```python
from build123d import *

# Parameters (mm, degrees)
SKETCH2_R           = 262.5
SKETCH2_R_2         = 75
SKETCH2_R_3         = 3.2639
SKETCH2_R_4         = 3.25
BOSS_EXTRUDE1_DEPTH = 6.35


with BuildPart() as part:
    # Sketch2 → Boss-Extrude1 (new body)
    with BuildSketch(Plane(origin=(0, 0, 0), x_dir=(1, 0, 0), z_dir=(0, 1, 0))):
        with Locations(Location((0, 0, 0), (0, 0, 270))):
            Circle(SKETCH2_R)
        with Locations(Location((0, 0, 0), (0, 0, 270))):
            Circle(SKETCH2_R_2, mode=Mode.SUBTRACT)
        with Locations(Location((-232.5, 12.7, 0), (0, 0, 270))):
            Circle(SKETCH2_R_3, mode=Mode.SUBTRACT)
        with Locations(Location((-172.5, 12.7, 0), (0, 0, 270))):
            Circle(SKETCH2_R_3, mode=Mode.SUBTRACT)
        with Locations(Location((-112.5, 12.7, 0), (0, 0, 270))):
            Circle(SKETCH2_R_3, mode=Mode.SUBTRACT)
        with Locations(Location((112.5, 12.7, 0), (0, 0, 270))):
            Circle(SKETCH2_R_3, mode=Mode.SUBTRACT)
        with Locations(Location((172.5, 12.7, 0), (0, 0, 270))):
            Circle(SKETCH2_R_3, mode=Mode.SUBTRACT)
        with Locations(Location((232.5, 12.7, 0), (0, 0, 270))):
            Circle(SKETCH2_R_3, mode=Mode.SUBTRACT)
        with Locations(Location((232.5, -12.7, 0), (0, 0, 270))):
            Circle(SKETCH2_R_3, mode=Mode.SUBTRACT)
        with Locations(Location((172.5, -12.7, 0), (0, 0, 270))):
            Circle(SKETCH2_R_3, mode=Mode.SUBTRACT)
        with Locations(Location((112.5, -12.7, 0), (0, 0, 270))):
            Circle(SKETCH2_R_3, mode=Mode.SUBTRACT)
        with Locations(Location((-112.5, -12.7, 0), (0, 0, 270))):
            Circle(SKETCH2_R_3, mode=Mode.SUBTRACT)
        with Locations(Location((-172.5, -12.7, 0), (0, 0, 270))):
            Circle(SKETCH2_R_3, mode=Mode.SUBTRACT)
        with Locations(Location((-232.5, -12.7, 0), (0, 0, 270))):
            Circle(SKETCH2_R_3, mode=Mode.SUBTRACT)
        with Locations(Location((-173.205080757, 100, 0), (0, 0, 270))):
            Circle(SKETCH2_R_4, mode=Mode.SUBTRACT)
        with Locations(Location((173.205080757, 100, 0), (0, 0, 270))):
            Circle(SKETCH2_R_4, mode=Mode.SUBTRACT)
        with Locations(Location((0, -200, 0), (0, 0, 270))):
            Circle(SKETCH2_R_4, mode=Mode.SUBTRACT)
        with BuildLine():
            Line((-43.05, 236.77567), (-43.05, 161.77567))
            ThreePointArc((-43.05, 161.77567), (-45.55, 159.27567), (-48.05, 161.77567))
            Line((-48.05, 161.77567), (-48.05, 236.77567))
            ThreePointArc((-48.05, 236.77567), (-45.55, 239.27567), (-43.05, 236.77567))
        make_face(mode=Mode.SUBTRACT)
        with BuildLine():
            Line((43.05, 236.77567), (43.05, 161.77567))
            ThreePointArc((43.05, 161.77567), (45.55, 159.27567), (48.05, 161.77567))
            Line((48.05, 161.77567), (48.05, 236.77567))
            ThreePointArc((48.05, 236.77567), (45.55, 239.27567), (43.05, 236.77567))
        make_face(mode=Mode.SUBTRACT)
        with BuildLine():
            Line((226.578745218, -81.105441367), (161.626839934, -43.605441367))
            ThreePointArc((161.626839934, -43.605441367), (160.711776425, -40.190377858), (164.126839934, -39.275314348))
            Line((164.126839934, -39.275314348), (229.078745218, -76.775314348))
            ThreePointArc((229.078745218, -76.775314348), (229.993808728, -80.190377858), (226.578745218, -81.105441367))
        make_face(mode=Mode.SUBTRACT)
        with BuildLine():
            Line((183.528745218, -155.670228633), (118.576839934, -118.170228633))
            ThreePointArc((118.576839934, -118.170228633), (115.161776425, -119.085292142), (116.076839934, -122.500355652))
            Line((116.076839934, -122.500355652), (181.028745218, -160.000355652))
            ThreePointArc((181.028745218, -160.000355652), (184.443808728, -159.085292142), (183.528745218, -155.670228633))
        make_face(mode=Mode.SUBTRACT)
        with BuildLine():
            Line((-183.528745218, -155.670228633), (-118.576839934, -118.170228633))
            ThreePointArc((-118.576839934, -118.170228633), (-115.161776425, -119.085292142), (-116.076839934, -122.500355652))
            Line((-116.076839934, -122.500355652), (-181.028745218, -160.000355652))
            ThreePointArc((-181.028745218, -160.000355652), (-184.443808728, -159.085292142), (-183.528745218, -155.670228633))
        make_face(mode=Mode.SUBTRACT)
        with BuildLine():
            Line((-226.578745218, -81.105441367), (-161.626839934, -43.605441367))
            ThreePointArc((-161.626839934, -43.605441367), (-160.711776425, -40.190377858), (-164.126839934, -39.275314348))
            Line((-164.126839934, -39.275314348), (-229.078745218, -76.775314348))
            ThreePointArc((-229.078745218, -76.775314348), (-229.993808728, -80.190377858), (-226.578745218, -81.105441367))
        make_face(mode=Mode.SUBTRACT)
    extrude(amount=BOSS_EXTRUDE1_DEPTH)


solid = part.part
```
Geometry check sheet. Reference: the model listing, model coordinates, mm. A direction names the side the tool comes from. Round coordinates to 2 decimals unless told otherwise and drop trailing zeros. Order: outer loops, then holes, each group sorted by start corner. A loop starts at its lowest first (then second) coordinate and runs counter-clockwise, first axis right, second up. Notation, with made-up numbers: (37, 64.25) - (53, 64.25) arc R15 ccw to (53, 87.25) - close; hole circle Ø5 at (67.5, 47.5). An arc over 180 degrees is marked (long way). Use a Markdown table: item, result. Add a question column.
(1) Depth check by flat-ended pin: pin 1 (1.5 mm diameter, centred on y = 2.5, z = -195.5, fed in from -X); pin 2 (3 mm diameter, centred on y = 2, z = -211.5, fed in from +X); pin 3 (6 mm diameter, centred on x = -173.21, z = -100, fed in from -Y); pin 4 (1.9 mm diameter, centred on y = 2, z = -191.5, fed in from +X). Enter the tip coordinate at first touch or a pass-through.
(2) Material ranges on line 1 along Z through (x, y) = (-231, 2.5); line 2 along X through (y, z) = (1, -187.5); line 3 along X through (y, z) = (1.25, -212.5), recorded low to high. Write a range as [from, to].
(3) Sectioned sample at B-B, the plane x = 149. Enter the section's corners in (y, z), and give its area (3 significant figures).
(4) Sectioned sample at A-A, the plane z = 0. Enter the section's corners in (x, y).
(5) Sectioned sample at D-D, the plane z = -141. Enter the section's corners in (x, y).
(6) Release check for a two-part mould opening along X. For faces 3 (the cylindrical face through (78.848, 3.131, 250.378)), 4 (the flat face through (196.148, 3.131, 57.763)), 5 (the flat face through (-194.56, 3.13, 62.62)), 6 (the flat face through (-55, 0, 55)) record: pulls with the +X half, pulls with the -X half, needs draft (parallel to the pull), parting line crosses it, or undercut.
(7) Sectioned sample at C-C, the plane y = 2.75. Count the separate pieces of the cut face and the enclosed holes in it, and give its area (3 significant figures).
(8) Tool access check on faces 1 (the flat face through (-151.507, 3.131, 137.183)), 2 (the flat face through (-55, 6.35, 55)). Record the directions out of +Z, -Z, +X, -X, +Y, -Y that give a thin tool (end or side, any length) a straight path to the whole face; none if there is none.
Answers below:
| question | item | result |
|---|---|---|
| 1 | pin 1 | x = -176.01 |
| 1 | pin 2 | x = 157.5 |
| 1 | pin 3 | through |
| 1 | pin 4 | x = 180.55 |
| 2 | line 1 | [-124.68, -15.6], [-9.8, 9.8], [15.6, 124.68] |
| 2 | line 2 | [-183.71, -48.05], [-43.05, 43.05], [48.05, 183.71] |
| 2 | line 3 | [-154.11, -48.05], [-43.05, 43.05], [48.05, 154.11] |
| 3 | outline | (0, -216.11) - (6.35, -216.11) - (6.35, 135.74) - (0, 135.74) - close; (0, 141.51) - (6.35, 141.51) - (6.35, 216.11) - (0, 216.11) - close |
| 3 | area | 2,710 mm² |
| 4 | outline | (-262.5, 0) - (-75, 0) - (-75, 6.35) - (-262.5, 6.35) - close; (75, 0) - (262.5, 0) - (262.5, 6.35) - (75, 6.35) - close |
| 5 | outline | (-221.42, 0) - (221.42, 0) - (221.42, 6.35) - (-221.42, 6.35) - close |
| 6 | face 3 | parting line crosses it |
| 6 | face 4 | undercut |
| 6 | face 5 | undercut |
| 6 | face 6 | needs draft |
| 7 | separate pieces | 1 |
| 7 | enclosed holes | 22 |
| 7 | area | 196,000 mm² |
| 8 | face 1 | +Y, -Y |
| 8 | face 2 | +Z, -Z, +X, -X, +Y |
